Autodesk Inventor part; units mm, degrees
ref_plane "YZ Plane" through (0, 0, 0) normal (1, 0, 0) x (0, 1, 0)
ref_plane "XZ Plane" through (0, 0, 0) normal (0, 1, 0) x (-1, 0, 0)
ref_plane "XY Plane" through (0, 0, 0) normal (0, 0, 1) x (1, 0, 0)
sketch "Sketch1" plane through (0, 0, 0) normal (0, 0, 1) x (1, 0, 0)
  circle A0 centre (0, 0) radius 1.95
  circle A1 centre (0, 0) radius 23.9014
  point P0 (0, 0)
  dimension "d0" = 47.8028
extrude "Extrusion1" add sketch "Sketch1" along normal blind 19.05
sketch "Sketch2" plane through (0, 0, 0) normal (0, 0, -1) x (-1, 0, 0)
  circle A0 centre (0, 0) radius 1.95
  circle A1 centre (0, 0) radius 23.9014
  circle A2 centre (0, 0) radius 12.7
  dimension "d3" = 25.4
extrude "Extrusion2" cut sketch "Sketch2" against normal blind 6.35 contours A1
sketch "Sketch3" plane through (0, 0, 19.05) normal (0, 0, 1) x (1, 0, 0)
  circle A0 centre (0, 0) radius 23.9014
  line L0 (-3.175, -17.5514) -> (3.175, -17.5514)
  line L1 (3.175, -17.5514) -> (3.175, -23.9014)
  line L2 (3.175, -23.9014) -> (-3.175, -23.9014)
  line L3 (-3.175, -23.9014) -> (-3.175, -17.5514)
  line L4 (0, 0) -> (0, -27.6264) construction
  point P0 (0, -17.5514)
  dimension "d6" = 6.35
  dimension "d7" = 6.35
extrude "Extrusion3" cut sketch "Sketch3" against normal blind 12.7 contours L3 L0 L1 A0 | A0 L2 L3 | L1 L2 A0 picked at (0, -19.6681)
pattern_circular "Circular Pattern1" count 10 over 360 about axis through (0, 0, 0) along (0, 0, 1) of "Extrusion3"
sketch "Sketch4" plane through (0, 0, 19.05) normal (0, 0, 1) x (1, 0, 0)
  arc A0 (-21.549, -10.3401) -> (-16.493, -17.2991) centre (0, 0) ccw
  circle A1 centre (0, 0) radius 23.9014
  circle A2 centre (0, 0) radius 25.6348
extrude "Extrusion4" add sketch "Sketch4" against normal blind 12.7
sketch "Sketch5" plane through (0, 0, 6.35) normal (0, 0, -1) x (-1, 0, 0)
  point P0 (-6.7, 20.6205)
hole "Hole1" at (6.7, 20.6205, 6.35) direction (0, 0, 1) diameter 3.175 depth 25.4 tip angle 118
pattern_circular "Circular Pattern2" count 10 over 360 about axis through (0, 0, 0) along (0, 0, 1) of "Hole1"
properties part number "driveWheel01" material "Wood (Maple)"
Check sheet for the modelled part. Datum: model origin and axes. Units: mm. Round coordinates to 2 decimals unless told otherwise and drop trailing zeros. Loops run counter-clockwise (first coordinate to the right, second up) from the corner with the lowest first, then second, coordinate; pieces in that order, holes last. Notation, with made-up numbers: (-35.75, 75.25) -> (9.25, 75.25) arc R20 cw to (9.25, 100.25) -> close; hole circle Ø2 at (52, 49). An arc over 180 degrees is marked (long way). Answer in a Markdown table with one row per item.
Q1. Sectioned sample at B-B on y = 6. Enter the section's corners in (x, z), then the cut area to 3 significant figures.
Data:
| item | result |
|---|---|
| outline | (-24.92, 6.35) -> (-23.14, 6.35) -> (-23.14, 19.05) -> (-24.92, 19.05) -> close; (-16.51, 6.35) -> (-11.19, 6.35) -> (-11.19, 0) -> (11.19, 0) -> (11.19, 6.35) -> (16.51, 6.35) -> (16.51, 19.05) -> (-16.51, 19.05) -> close; (23.14, 6.35) -> (24.92, 6.35) -> (24.92, 19.05) -> (23.14, 19.05) -> close |
| area | 607 mm^2 |
Q2. Sectioned sample at D-D on x = -6.7. Enter the section's corners in (y, z).
Data:
| item | result |
|---|---|
| outline | (-24.74, 6.35) -> (-22.21, 6.35) -> (-22.21, 19.05) -> (-24.74, 19.05) -> close; (-19.03, 6.35) -> (-10.79, 6.35) -> (-10.79, 0) -> (10.79, 0) -> (10.79, 6.35) -> (19.03, 6.35) -> (19.03, 19.05) -> (-19.03, 19.05) -> close; (22.21, 6.35) -> (24.74, 6.35) -> (24.74, 19.05) -> (22.21, 19.05) -> close |
Q3. Sectioned sample at C-C on z = 3.5. Enter the section's corners in (x, y), then the cut area to 3 significant figures.
Data:
| item | result |
|---|---|
| outline | circle Ø25.4 at (0, 0); hole circle Ø3.9 at (0, 0) |
| area | 495 mm^2 |
Q4. Thickness scan on L1, parallel to Y at x = 0, z = 11; L2, parallel to X at y = -20, z = 8 (3 decimals); L3, parallel to Y at x = -15, z = 8.75. Record the ranges inside material, lowest first.
Data:
| item | result |
|---|---|
| L1 | y = -25.63 to -23.9, -17.55 to -1.95, 1.95 to 17.55, 23.9 to 25.63 |
| L2 | x = -16.036 to -13.087, -10.606 to -8.161, -5.239 to -3.175, 3.175 to 5.239, 8.161 to 10.606, 13.087 to 16.036 |
| L3 | y = -20.79 to -18.61, -15.24 to 15.24, 18.61 to 20.79 |
Q5. Sectioned sample at A-A on x = 0. Enter the section's corners in (y, z), then the cut area to 3 significant figures.
Data:
| item | result |
|---|---|
| outline | (-25.63, 6.35) -> (-23.9, 6.35) -> (-23.9, 19.05) -> (-25.63, 19.05) -> close; (-17.55, 6.35) -> (-12.7, 6.35) -> (-12.7, 0) -> (-1.95, 0) -> (-1.95, 19.05) -> (-17.55, 19.05) -> close; (1.95, 0) -> (12.7, 0) -> (12.7, 6.35) -> (17.55, 6.35) -> (17.55, 19.05) -> (1.95, 19.05) -> close; (23.9, 6.35) -> (25.63, 6.35) -> (25.63, 19.05) -> (23.9, 19.05) -> close |
| area | 577 mm^2 |
Q6. Release check for a two-part mould opening along X. For faces 1 (the face through (0, -5, 19.05)), 2 (the face through (0, 23.9, 12.8)) record: released by +X, released by -X, zero draft, split by the parting line, or undercut.
Data:
| item | result |
|---|---|
| face 1 | zero draft |
| face 2 | undercut |
Q7. Go/stop test with flat-tipped pins: P1, Ø7, axis at y = -21.5, z = 11, coming from the -X side; P2, Ø6, axis at x = 7.5, y = 16.5, coming from the -Z side; P3, Ø10, axis at x = -8, z = 7.5, coming from the -Y side. Record where each tip stops, or that it passes through.
Data:
| item | result |
|---|---|
| P1 | stops at x = -18.25 |
| P2 | stops at z = 6.35 |
| P3 | stops at y = -25.46 |
